Autodesk Inventor part; units mm, degrees
ref_plane "YZ Plane" through (0, 0, 0) normal (1, 0, 0) x (0, 1, 0)
ref_plane "XZ Plane" through (0, 0, 0) normal (0, 1, 0) x (-1, 0, 0)
ref_plane "XY Plane" through (0, 0, 0) normal (0, 0, 1) x (1, 0, 0)
sketch "Sketch1" plane through (0, 0, 0) normal (1, 0, 0) x (0, 1, 0)
  line L0 (0, 0) -> (13, 0)
  line L1 (13, 0) -> (13, -27)
  line L2 (13, -27) -> (0, -27)
  line L3 (0, -27) -> (0, 0)
  dimension "d0" = 13
  dimension "d1" = 27
extrude "Extrusion1" add sketch "Sketch1" along normal blind 40
sketch "Sketch2" plane through (40, 0, 0) normal (1, 0, 0) x (0, 0, -1)
  line L0 (27, 0) -> (27, 13)
  line L1 (27, 0) -> (33, 0)
  line L2 (33, 0) -> (33, 38)
  line L3 (33, 38) -> (27, 38)
  line L4 (27, 38) -> (27, 0)
  point P0 (0, 0)
  dimension "d4" = 6
  dimension "d5" = 38
extrude "Extrusion2" add sketch "Sketch2" against normal blind 40
sketch "Sketch3" plane through (0, 13, 0) normal (0, 1, 0) x (1, 0, 0)
  line L0 (40, 27) -> (40, 0) construction
  line L1 (40, 0) -> (35, 0) construction
  line L2 (0, 0) -> (40, 0) construction
  line L3 (35, 0) -> (35, 5) construction
  line L4 (35, 5) -> (35, 15) construction
  line L5 (35, 5) -> (9.6, 5) construction
  line L6 (35, 5) -> (35, 15) construction
  line L7 (36.65, 5) -> (36.65, 15)
  line L8 (33.35, 15) -> (33.35, 5)
  arc A0 (33.35, 5) -> (36.65, 5) centre (35, 5) ccw
  arc A1 (36.65, 15) -> (33.35, 15) centre (35, 15) ccw
  line L9 (9.6, 0) -> (9.6, 5) construction
  line L10 (9.6, 5) -> (9.6, 15) construction
  line L11 (9.6, 5) -> (-15.8, 5) construction
  line L12 (9.6, 5) -> (9.6, 15) construction
  line L13 (11.25, 5) -> (11.25, 15)
  line L14 (7.95, 15) -> (7.95, 5)
  arc A2 (7.95, 5) -> (11.25, 5) centre (9.6, 5) ccw
  arc A3 (11.25, 15) -> (7.95, 15) centre (9.6, 15) ccw
  point P0 (35, 10)
  point P1 (9.6, 10)
  dimension "d8" = 5
  dimension "d9" = 5
  dimension "d10" = 10
  dimension "d11" = 25.4
  dimension "d12" = 3.3
  dimension "d13" = 5
  dimension "d14" = 10
  dimension "d15" = 25.4
  dimension "d16" = 3.3
extrude "Extrusion3" cut sketch "Sketch3" against normal blind 40
sketch "Sketch4" plane through (0, 13, 0) normal (0, 1, 0) x (1, 0, 0)
  point P0 (0, 0)
sketch "Sketch7" plane through (40, 13, -27) normal (0, 0, 1) x (1, 0, 0)
  line L0 (0, 25) -> (0, 0)
  line L1 (-40, 0) -> (0, 0)
  line L2 (0, 25) -> (-20, 25)
  line L3 (-20, 25) -> (-20, 0)
  line L4 (-20, 0) -> (0, 0)
  line L5 (0, 0) -> (0, 25)
  point P0 (-40, -13)
extrude "Extrusion6" cut sketch "Sketch7" against normal blind 45.275
sketch "Sketch9" plane through (0, 0, 0) normal (-1, 0, 0) x (0, 0, 1)
  line L0 (0, 0) -> (0, 3.6) construction
  line L1 (0, 13) -> (0, 0) construction
  line L2 (0, 3.6) -> (-18, 3.6)
  line L3 (-18, 3.6) -> (-18, 13)
  line L4 (-18, 13) -> (0, 13)
  line L5 (0, 13) -> (0, 3.6)
  dimension "d58" = 3.6
  dimension "d59" = 18
extrude "Extrusion8" cut sketch "Sketch9" against normal blind 50.325
sketch "Sketch10" plane through (40, 0, -33) normal (0, 0, -1) x (-1, 0, 0)
  point P0 (40, 0)
sketch "Sketch8" plane through (0, 13, -27) normal (0, 1, 0) x (1, 0, 0)
  line L0 (0, 0) -> (20, 0) construction
  line L1 (0, 0) -> (2.5, 0) construction
  line L2 (2.5, 0) -> (14.5, 0)
  line L3 (14.5, 0) -> (14.5, -10)
  line L4 (14.5, -10) -> (2.5, -10)
  line L5 (2.5, -10) -> (2.5, 0)
  point P0 (0, -27)
  point P1 (26.7625, 0)
  dimension "d53" = 2.5
  dimension "d54" = 12
  dimension "d55" = 10
extrude "Extrusion7" cut sketch "Sketch8" against normal blind 1.5
sketch "Sketch11" plane through (0, 0, 0) normal (-1, 0, 0) x (0, 0, 1)
  line L0 (0, 3.6) -> (-18, 3.6)
  line L1 (-18, 3.6) -> (-18, 13)
  line L2 (-27, 13) -> (-18, 13)
  line L3 (-27, 13) -> (-27, 38)
  line L4 (-27, 38) -> (-33, 38)
  line L5 (-33, 38) -> (-33, 0)
  line L6 (0, 0) -> (-33, 0)
  line L7 (0, 3.6) -> (0, 0)
extrude "Extrusion9" add sketch "Sketch11" along normal blind 9.05
sketch "Sketch6" plane through (40, 13, -27) normal (0, 0, 1) x (1, 0, 0)
  line L0 (-40, 0) -> (0, 0) construction
  line L1 (-47.2016, 0) -> (-47.2016, 2.3001) construction
  line L2 (-40, 25) -> (-40, -13) construction
  line L3 (-47.2016, 2.3001) -> (-13.7954, 2.3001) construction
  line L4 (-47.2016, 2.3001) -> (-47.2016, 19.8001) construction
  line L5 (-47.2016, 19.8001) -> (-14.7386, 19.8001) construction
  line L6 (-47.2016, 2.3001) -> (-43.2016, 2.3001) construction
  line L7 (-43.2016, 2.3001) -> (-43.2016, 19.8001) construction
  line L8 (-43.2016, 19.8001) -> (-31.2016, 19.8001) construction
  line L9 (-43.2016, 2.3001) -> (-31.2016, 2.3001) construction
  line L10 (-43.2016, 19.8001) -> (-31.2016, 19.8001) construction
  line L11 (-43.2016, 18.0501) -> (-31.2016, 18.0501)
  line L12 (-31.2016, 21.5501) -> (-43.2016, 21.5501)
  arc A0 (-43.2016, 21.5501) -> (-43.2016, 18.0501) centre (-43.2016, 19.8001) ccw
  arc A1 (-31.2016, 18.0501) -> (-31.2016, 21.5501) centre (-31.2016, 19.8001) ccw
  line L13 (-43.2016, 2.3001) -> (-31.2016, 2.3001) construction
  line L14 (-43.2016, 0.5501) -> (-31.2016, 0.5501)
  line L15 (-31.2016, 4.0501) -> (-43.2016, 4.0501)
  arc A2 (-43.2016, 4.0501) -> (-43.2016, 0.5501) centre (-43.2016, 2.3001) ccw
  arc A3 (-31.2016, 0.5501) -> (-31.2016, 4.0501) centre (-31.2016, 2.3001) ccw
  point P0 (-37.2016, 19.8001)
  point P1 (-37.2016, 2.3001)
  dimension "d28" = 7.56
  dimension "d29" = 17.5
  dimension "d30" = 4
  dimension "d31" = 12
  dimension "d32" = 12
  dimension "d33" = 3.5
  dimension "d34" = 3.5
extrude "Extrusion5" cut sketch "Sketch6" against normal blind 35.6875
sketch "Sketch13" plane through (2.5, 13, -18) normal (0, 1, 0) x (1, 0, 0)
  line L0 (-11.55, 0) -> (37.5, 0)
  line L1 (6.2984, 9) -> (-5.7016, 9)
  line L2 (-8.4479, 0) -> (0.0285, 0)
  line L3 (0.0285, 0) -> (0.0285, 9)
  line L4 (0.0285, 9) -> (-8.4479, 9)
  line L5 (-8.4479, 9) -> (-8.4479, 0)
  point P0 (-2.5, -18)
  point P1 (5.45, 0)
  point P2 (0.0285, 0)
  point P3 (-5.7016, 9)
extrude "Extrusion10" cut sketch "Sketch13" against normal up to surface (1.5 mm away)
chamfer "Chamfer5" distance 8.35 angle 45 1 edges at (40, 13, -25.5)
sketch "Sketch14" plane through (20, 13, -27) normal (1, 0, 0) x (0, 0, -1)
  line L0 (6, 25) -> (6, 0)
  line L1 (0, 25) -> (6, 25)
  line L2 (0, 0) -> (0, 25)
  line L3 (0, 0) -> (6, 0)
  point P0 (-27, -13)
extrude "Extrusion11" cut sketch "Sketch14" against normal blind 5.2375
chamfer "Chamfer6" distance 8.35 angle 45 1 edges at (14.7625, 13, -30)
chamfer "Chamfer7" distance 2 angle 45 2 edges at (14.7625, 38, -30) (-9.05, 38, -30)
chamfer "Chamfer8" distance 2 angle 45 4 edges at (40, 1.8, 0) (-9.05, 1.8, 0) (40, 2.325, -33) (-9.05, 18, -33)
properties part number "Motor Mount v2"
Geometry check sheet. Reference: the model listing, model coordinates, mm. A direction names the side the tool comes from. Coordinates: 2 decimals unless noted, no trailing zeros. Order: outer loops, then holes, each group sorted by start corner. A loop starts at its lowest first (then second) coordinate and runs counter-clockwise, first axis right, second up. Notation, with made-up numbers: M 22.25,39 L 73.25,39 A26 ccw 73.25,72 Z; hole C 22.5,12 d10. An arc over 180 degrees is marked long. Use CSV: the item, a comma, the result in double quotes.
Item 1: Cross-section at C-C on x = 35. Record the cut outline in (y, z).
Returned:
outline,"M 0,-33 L 9.65,-33 L 9.65,-18 L 3.6,-18 L 3.6,-16.65 L 0,-16.65 Z; M 0,-3.35 L 3.6,-3.35 L 3.6,0 L 0,0 Z"
Item 2: Cross-section at A-A on x = -0.5. Record the cut outline in (y, z).
Returned:
outline,"M 0,-33 L 13.55,-33 L 13.55,-27 L 11.5,-27 L 11.5,-18 L 3.6,-18 L 3.6,0 L 0,0 Z; M 17.05,-33 L 31.05,-33 L 31.05,-27 L 17.05,-27 Z; M 34.55,-33 L 38,-33 L 38,-27 L 34.55,-27 Z"
Item 3: Mould release check, pull along X, two halves, no side actions. Record for faces 1 (the flat face through (16, 3.6, -9)), 2 (the flat face through (39, 2, -1)), 3 (the cylindrical face through (10.548, 15.262, -29.958)), 4 (the cylindrical face through (9.64, 1.83, -16.65)): pulls with the +X half, pulls with the -X half, needs draft (parallel to the pull), parting line crosses it, or undercut.
Returned:
face 1,"needs draft"
face 2,"pulls with the +X half"
face 3,"undercut"
face 4,"undercut"
Item 4: Thickness scan on line 1 along Y through (x, z) = (12, -4.5); line 2 along Z through (x, y) = (2.5, 30); line 3 along Y through (x, z) = (21, -24). Record the ranges inside material, lowest first.
Returned:
line 1,"y = 0 to 3.6"
line 2,"z = -33 to -27"
line 3,"y = 0 to 13"
Item 5: Cross-section at B-B on z = -6.5. Record the cut outline in (x, y), then the cut area to 3 significant figures.
Returned:
outline,"M -9.05,0 L 7.95,0 L 7.95,3.6 L -9.05,3.6 Z; M 11.25,0 L 33.35,0 L 33.35,3.6 L 11.25,3.6 Z; M 36.65,0 L 40,0 L 40,3.6 L 36.65,3.6 Z"
area,"153 mm2"
Item 6: Gauge pin test, flat ends, axial feed: pin 1 Ø1.6 at (x, z) = (-8, -22.5) entering from +Y; pin 2 Ø12 at (x, y) = (-1.5, 9) entering from +Z; pin 3 Ø8 at (x, y) = (13.5, 25) entering from +Z; pin 4 Ø8 at (y, z) = (14.5, -19.5) entering from +X. Record the tip position at first contact, or that the pin passes through.
Returned:
pin 1,"stops at y = 13"
pin 2,"stops at z = 0"
pin 3,"stops at z = -27"
pin 4,"stops at x = 34.15"
Item 7: Tool access check on faces 5 (the flat face through (3, 34.55, -30)), 6 (the cylindrical face through (35.04, 1.83, -16.65)), 7 (the flat face through (14.762, 29, -30)). Record the directions out of +Z, -Z, +X, -X, +Y, -Y that give a thin tool (end or side, any length) a straight path to the whole face; none if there is none.
Returned:
face 5,"+Z, -Z"
face 6,"+Y, -Y"
face 7,"+Z, -Z, +X, +Y"
Item 8: Cross-section at D-D on y = 3. Record the cut outline in (x, z), then the cut area to 3 significant figures.
Returned:
outline,"M -9.05,-31 L -7.05,-33 L 38,-33 L 40,-31 L 40,-2 L 38,0 L -7.05,0 L -9.05,-2 Z; hole M 7.95,-15 A1.65 ccw 11.25,-15 L 11.25,-5 A1.65 ccw 7.95,-5 Z; hole M 33.35,-15 A1.65 ccw 36.65,-15 L 36.65,-5 A1.65 ccw 33.35,-5 Z"
area,"1,530 mm2"
